The figure shows three views and two pictorial views of one solid part (mm, origin at its lowest corner). Answer the questions. Coordinates: 2 decimals unless noted, no trailing zeros. Order: outer loops, then holes, each group sorted by start corner. A loop starts at its lowest first (then second) coordinate and runs counter-clockwise, first axis right, second up. Notation, with made-up numbers: M 85,35 L 92,35 A14 ccw 92,39 Z; hole C -0.75,-28.75 d1. An arc over 180 degrees is marked long. Use a Markdown table: item, result.
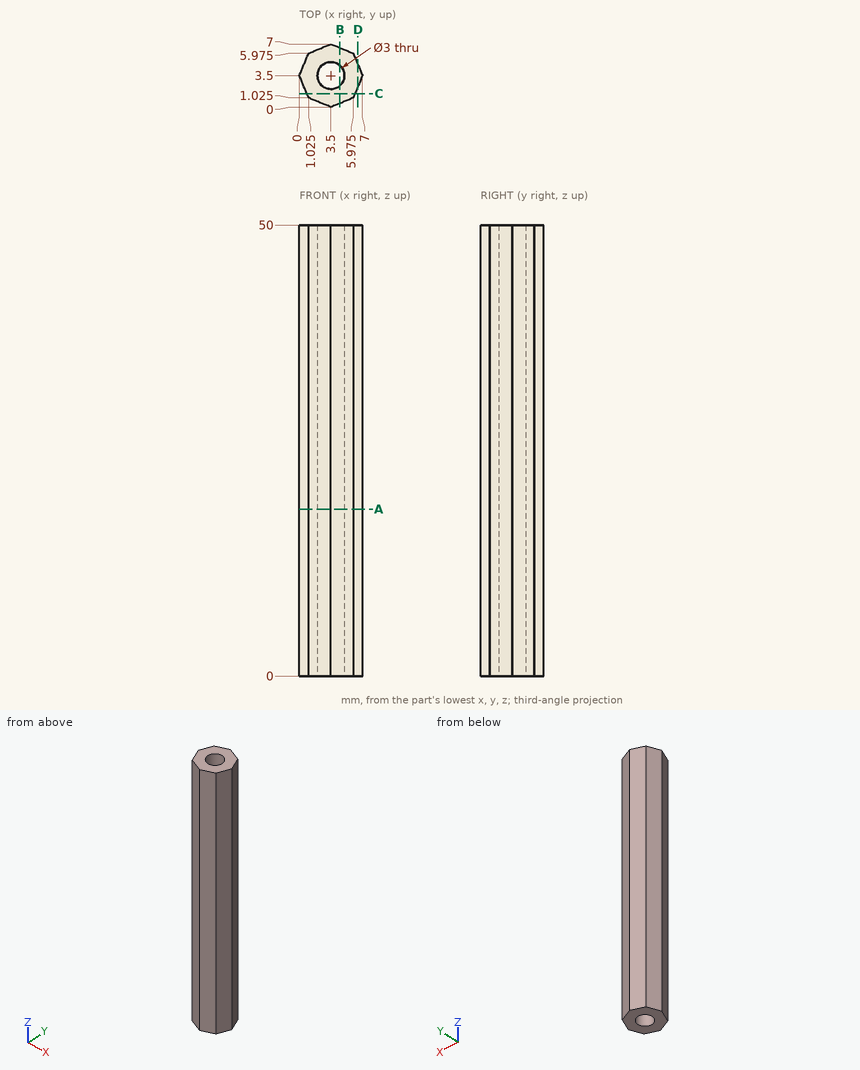
1. Find the intervals of material crossed by probe 1 along Y at (x, z) = (4, 35); probe 2 along X at (y, z) = (4.5, 45); probe 3 along Y at (x, z) = (1.5, 23), in increasing order.
Answers below:
| item | result |
|---|---|
| probe 1 | 0.21 to 2.09, 4.91 to 6.79 |
| probe 2 | 0.41 to 2.38, 4.62 to 6.59 |
| probe 3 | 0.83 to 6.17 |
2. Section A-A on z = 18.5 is taken. Determine the outline of the cut face in (x, y) (3 decimals).
Answers below:
| item | result |
|---|---|
| outline | M 0,3.5 L 1.025,1.025 L 3.5,0 L 5.975,1.025 L 7,3.5 L 5.975,5.975 L 3.5,7 L 1.025,5.975 Z; hole C 3.5,3.5 d3 |
3. Section D-D on x = 6.5 is taken. Determine the outline of the cut face in (y, z).
Answers below:
| item | result |
|---|---|
| outline | M 2.29,0 L 4.71,0 L 4.71,50 L 2.29,50 Z |
4. Section C-C on y = 1.5 is taken. Determine the outline of the cut face in (x, z), then the cut area to 3 significant figures.
Answers below:
| item | result |
|---|---|
| outline | M 0.83,0 L 6.17,0 L 6.17,50 L 0.83,50 Z |
| area | 267 mm² |
5. Section B-B on x = 4.5 is taken. Determine the outline of the cut face in (y, z), then the cut area to 3 significant figures.
Answers below:
| item | result |
|---|---|
| outline | M 0.41,0 L 2.38,0 L 2.38,50 L 0.41,50 Z; M 4.62,0 L 6.59,0 L 6.59,50 L 4.62,50 Z |
| area | 197 mm² |
6. Flat-ended cylindrical pins translate along their axes: P1, Ø1, axis at y = 1.5, z = 24.5, coming from the +X side; P2, Ø1.5, axis at x = 2.5, z = 42, coming from the -Y side; P3, Ø1.5, axis at x = 5.5, z = 27.5, coming from the +Y side. Find the tip coordinate at first contact, or state that the pin passes through.
Answers below:
| item | result |
|---|---|
| P1 | x = 6.38 |
| P2 | y = 0.1 |
| P3 | y = 6.48 |
